Geometry check sheet. Reference: the model listing, model coordinates, mm. Face numbers are marked on the shaded views. Coordinates: 2 decimals unless noted, no trailing zeros. Write item = value, one per line. Start each with the question number.
from build123d import *
from OCP.BRepFilletAPI import BRepFilletAPI_MakeChamfer

# Parameters (mm, degrees)
SKETCH1_R           = 5.25
BOSS_EXTRUDE1_DEPTH = 20
SKETCH1_3_R         = 1.5
BOSS_EXTRUDE2_DEPTH = 17
FILLET1_R           = 15
CHAMFER1_SIZE       = 8.660254038
CHAMFER1_SIZE_2     = 5


with BuildPart() as part:
    # Sketch1 → Boss-Extrude1 (new body)
    # profile 1 of 7: a face of its own
    with BuildSketch(Plane(origin=(0, 0, 0), x_dir=(1, 0, 0), z_dir=(0, 1, 0))):
        with BuildLine():
            Line((-17.320508076, 0), (-12.990381057, 7.5))
            ThreePointArc((-12.990381057, 7.5), (-25.980762114, 0), (-12.990381057, -7.5))
            Line((-12.990381057, -7.5), (-17.320508076, 0))
        make_face()
    # profile 2 of 7: a face of its own
    with BuildSketch(Plane(origin=(0, 0, 0), x_dir=(1, 0, 0), z_dir=(0, 1, 0))):
        Polygon((17.320508076, 0), (8.660254038, 15), (-8.660254038, 15), (-17.320508076, 0), (-8.660254038, -15), (8.660254038, -15), align=None)
        with Locations(Location((0, 0, 0), (0, 0, 270))):
            Circle(SKETCH1_R, mode=Mode.SUBTRACT)
        Polygon((1.443375673, -5.5), (-1.443375673, -5.5), (-2.886751346, -8), (-1.443375673, -10.5), (1.443375673, -10.5), (2.886751346, -8), align=None, mode=Mode.SUBTRACT)
        Polygon((8, 2.886751346), (5.5, 1.443375673), (5.5, -1.443375673), (8, -2.886751346), (10.5, -1.443375673), (10.5, 1.443375673), align=None, mode=Mode.SUBTRACT)
        Polygon((2.886751346, 8), (1.443375673, 10.5), (-1.443375673, 10.5), (-2.886751346, 8), (-1.443375673, 5.5), (1.443375673, 5.5), align=None, mode=Mode.SUBTRACT)
        Polygon((-8, 2.886751346), (-10.5, 1.443375673), (-10.5, -1.443375673), (-8, -2.886751346), (-5.5, -1.443375673), (-5.5, 1.443375673), align=None, mode=Mode.SUBTRACT)
    # profile 3 of 7: a face of its own
    with BuildSketch(Plane(origin=(0, 0, 0), x_dir=(1, 0, 0), z_dir=(0, 1, 0))):
        with BuildLine():
            Line((-12.990381057, 7.5), (-8.660254038, 15))
            Line((-8.660254038, 15), (0, 15))
            ThreePointArc((0, 15), (-12.990381057, 22.5), (-12.990381057, 7.5))
        make_face()
    # profile 4 of 7: a face of its own
    with BuildSketch(Plane(origin=(0, 0, 0), x_dir=(1, 0, 0), z_dir=(0, 1, 0))):
        with BuildLine():
            ThreePointArc((12.990381057, 7.5), (12.990381057, 22.5), (0, 15))
            Line((0, 15), (8.660254038, 15))
            Line((8.660254038, 15), (12.990381057, 7.5))
        make_face()
    # profile 5 of 7: a face of its own
    with BuildSketch(Plane(origin=(0, 0, 0), x_dir=(1, 0, 0), z_dir=(0, 1, 0))):
        with BuildLine():
            ThreePointArc((12.990381057, -7.5), (25.980762114, 0), (12.990381057, 7.5))
            Line((12.990381057, 7.5), (17.320508076, 0))
            Line((17.320508076, 0), (12.990381057, -7.5))
        make_face()
    # profile 6 of 7: a face of its own
    with BuildSketch(Plane(origin=(0, 0, 0), x_dir=(1, 0, 0), z_dir=(0, 1, 0))):
        with BuildLine():
            Line((8.660254038, -15), (0, -15))
            ThreePointArc((0, -15), (12.990381057, -22.5), (12.990381057, -7.5))
            Line((12.990381057, -7.5), (8.660254038, -15))
        make_face()
    # profile 7 of 7: a face of its own
    with BuildSketch(Plane(origin=(0, 0, 0), x_dir=(1, 0, 0), z_dir=(0, 1, 0))):
        with BuildLine():
            Line((-8.660254038, -15), (-12.990381057, -7.5))
            ThreePointArc((-12.990381057, -7.5), (-12.990381057, -22.5), (0, -15))
            Line((0, -15), (-8.660254038, -15))
        make_face()
    extrude(amount=BOSS_EXTRUDE1_DEPTH)

    # Sketch1<3> → Boss-Extrude2 (add)
    # profile 1 of 4: a face of its own
    with BuildSketch(Plane(origin=(0, 0, 0), x_dir=(1, 0, 0), z_dir=(0, 1, 0))):
        Polygon((-8.977463126, 2.322412747), (-10.5, 1.443375673), (-10.5, -1.443375673), (-8.977463126, -2.322412747), (-8, -2.886751346), (-5.5, -1.443375673), (-5.5, 1.443375673), (-8, 2.886751346), align=None)
        with Locations(Location((-8, 0, 0), (0, 0, 90))):
            Circle(SKETCH1_3_R, mode=Mode.SUBTRACT)
    # profile 2 of 4: a face of its own
    with BuildSketch(Plane(origin=(0, 0, 0), x_dir=(1, 0, 0), z_dir=(0, 1, 0))):
        Polygon((2.128194303, 9.313859338), (1.443375673, 10.5), (-1.443375673, 10.5), (-2.128194303, 9.313859338), (-2.886751346, 8), (-1.443375673, 5.5), (1.443375673, 5.5), (2.886751346, 8), align=None)
        with Locations(Location((0, 8, 0), (0, 0, 90))):
            Circle(SKETCH1_3_R, mode=Mode.SUBTRACT)
    # profile 3 of 4: a face of its own
    with BuildSketch(Plane(origin=(0, 0, 0), x_dir=(1, 0, 0), z_dir=(0, 1, 0))):
        Polygon((8, 2.886751346), (5.5, 1.443375673), (5.5, -1.443375673), (8, -2.886751346), (8.977463126, -2.322412747), (10.5, -1.443375673), (10.5, 1.443375673), (8.977463126, 2.322412747), align=None)
        with Locations(Location((8, 0, 0), (0, 0, 90))):
            Circle(SKETCH1_3_R, mode=Mode.SUBTRACT)
    # profile 4 of 4: a face of its own
    with BuildSketch(Plane(origin=(0, 0, 0), x_dir=(1, 0, 0), z_dir=(0, 1, 0))):
        Polygon((1.443375673, -5.5), (-1.443375673, -5.5), (-2.886751346, -8), (-2.128194303, -9.313859338), (-1.443375673, -10.5), (1.443375673, -10.5), (2.128194303, -9.313859338), (2.886751346, -8), align=None)
        with Locations(Location((0, -8, 0), (0, 0, 90))):
            Circle(SKETCH1_3_R, mode=Mode.SUBTRACT)
    extrude(amount=BOSS_EXTRUDE2_DEPTH)

    # Fillet1
    fillet1_edges = [part.edges().sort_by_distance(p)[0] for p in [
        (12.990381057, 10, 7.5),
        (0, 10, 15),
        (-12.990381057, 10, 7.5),
        (-12.990381057, 10, -7.5),
        (0, 10, -15),
        (12.990381057, 10, -7.5),
    ]]
    fillet(fillet1_edges, radius=FILLET1_R)

    # Chamfer1
    chamfer1_edges_1 = [part.edges().sort_by_distance(p)[0] for p in [
        (12.990381057, 20, 22.5),
    ]]
    chamfer1_side_1 = [part.faces().sort_by_distance(p)[0] for p in [
        (12.940381057, 20, 22.41339746),
    ]]
    chamfer1_edges_2 = [part.edges().sort_by_distance(p)[0] for p in [
        (-12.990381057, 20, 22.5),
    ]]
    chamfer1_side_2 = [part.faces().sort_by_distance(p)[0] for p in [
        (-12.940381057, 20, 22.41339746),
    ]]
    chamfer1_edges_3 = [part.edges().sort_by_distance(p)[0] for p in [
        (25.980762114, 20, 0),
    ]]
    chamfer1_side_3 = [part.faces().sort_by_distance(p)[0] for p in [
        (25.880762114, 20, 0),
    ]]
    chamfer1_edges_4 = [part.edges().sort_by_distance(p)[0] for p in [
        (12.990381057, 20, -22.5),
    ]]
    chamfer1_side_4 = [part.faces().sort_by_distance(p)[0] for p in [
        (12.940381057, 20, -22.41339746),
    ]]
    chamfer1_edges_5 = [part.edges().sort_by_distance(p)[0] for p in [
        (-12.990381057, 20, -22.5),
    ]]
    chamfer1_side_5 = [part.faces().sort_by_distance(p)[0] for p in [
        (-12.940381057, 20, -22.41339746),
    ]]
    chamfer1_edges_6 = [part.edges().sort_by_distance(p)[0] for p in [
        (-25.980762114, 20, 0),
    ]]
    chamfer1_side_6 = [part.faces().sort_by_distance(p)[0] for p in [
        (-25.980762114, 19.9, 0),
    ]]
    chamfer1_edges_7 = [part.edges().sort_by_distance(p)[0] for p in [
        (0, 20, 22.018347375),
    ]]
    chamfer1_side_7 = [part.faces().sort_by_distance(p)[0] for p in [
        (0, 20, 21.918347375),
    ]]
    chamfer1_edges_8 = [part.edges().sort_by_distance(p)[0] for p in [
        (19.068448176, 20, 11.009173688),
    ]]
    chamfer1_side_8 = [part.faces().sort_by_distance(p)[0] for p in [
        (18.981845636, 20, 10.959173688),
    ]]
    chamfer1_edges_9 = [part.edges().sort_by_distance(p)[0] for p in [
        (19.068448176, 20, -11.009173688),
    ]]
    chamfer1_side_9 = [part.faces().sort_by_distance(p)[0] for p in [
        (18.981845636, 20, -10.959173688),
    ]]
    chamfer1_edges_10 = [part.edges().sort_by_distance(p)[0] for p in [
        (0, 20, -22.018347375),
    ]]
    chamfer1_side_10 = [part.faces().sort_by_distance(p)[0] for p in [
        (0, 20, -21.918347375),
    ]]
    chamfer1_edges_11 = [part.edges().sort_by_distance(p)[0] for p in [
        (-19.068448176, 20, -11.009173688),
    ]]
    chamfer1_side_11 = [part.faces().sort_by_distance(p)[0] for p in [
        (-19.068448176, 19.9, -11.009173688),
    ]]
    chamfer1_edges_12 = [part.edges().sort_by_distance(p)[0] for p in [
        (-19.068448176, 20, 11.009173688),
    ]]
    chamfer1_side_12 = [part.faces().sort_by_distance(p)[0] for p in [
        (-19.068448176, 19.9, 11.009173688),
    ]]
    chamfer1 = BRepFilletAPI_MakeChamfer(part.part.solid().wrapped)
    for e in chamfer1_edges_1:
        chamfer1.Add(CHAMFER1_SIZE - 0.0001, CHAMFER1_SIZE_2 - 0.0001, e.wrapped, chamfer1_side_1[0].wrapped)
    for e in chamfer1_edges_2:
        chamfer1.Add(CHAMFER1_SIZE - 0.0001, CHAMFER1_SIZE_2 - 0.0001, e.wrapped, chamfer1_side_2[0].wrapped)
    for e in chamfer1_edges_3:
        chamfer1.Add(CHAMFER1_SIZE - 0.0001, CHAMFER1_SIZE_2 - 0.0001, e.wrapped, chamfer1_side_3[0].wrapped)
    for e in chamfer1_edges_4:
        chamfer1.Add(CHAMFER1_SIZE - 0.0001, CHAMFER1_SIZE_2 - 0.0001, e.wrapped, chamfer1_side_4[0].wrapped)
    for e in chamfer1_edges_5:
        chamfer1.Add(CHAMFER1_SIZE - 0.0001, CHAMFER1_SIZE_2 - 0.0001, e.wrapped, chamfer1_side_5[0].wrapped)
    for e in chamfer1_edges_6:
        chamfer1.Add(CHAMFER1_SIZE_2 - 0.0001, CHAMFER1_SIZE - 0.0001, e.wrapped, chamfer1_side_6[0].wrapped)
    for e in chamfer1_edges_7:
        chamfer1.Add(CHAMFER1_SIZE - 0.0001, CHAMFER1_SIZE_2 - 0.0001, e.wrapped, chamfer1_side_7[0].wrapped)
    for e in chamfer1_edges_8:
        chamfer1.Add(CHAMFER1_SIZE - 0.0001, CHAMFER1_SIZE_2 - 0.0001, e.wrapped, chamfer1_side_8[0].wrapped)
    for e in chamfer1_edges_9:
        chamfer1.Add(CHAMFER1_SIZE - 0.0001, CHAMFER1_SIZE_2 - 0.0001, e.wrapped, chamfer1_side_9[0].wrapped)
    for e in chamfer1_edges_10:
        chamfer1.Add(CHAMFER1_SIZE - 0.0001, CHAMFER1_SIZE_2 - 0.0001, e.wrapped, chamfer1_side_10[0].wrapped)
    for e in chamfer1_edges_11:
        chamfer1.Add(CHAMFER1_SIZE_2 - 0.0001, CHAMFER1_SIZE - 0.0001, e.wrapped, chamfer1_side_11[0].wrapped)
    for e in chamfer1_edges_12:
        chamfer1.Add(CHAMFER1_SIZE_2 - 0.0001, CHAMFER1_SIZE - 0.0001, e.wrapped, chamfer1_side_12[0].wrapped)
    add(Compound.cast(chamfer1.Shape()), mode=Mode.REPLACE)  # a hair under: the kernel refuses the full size


solid = part.part
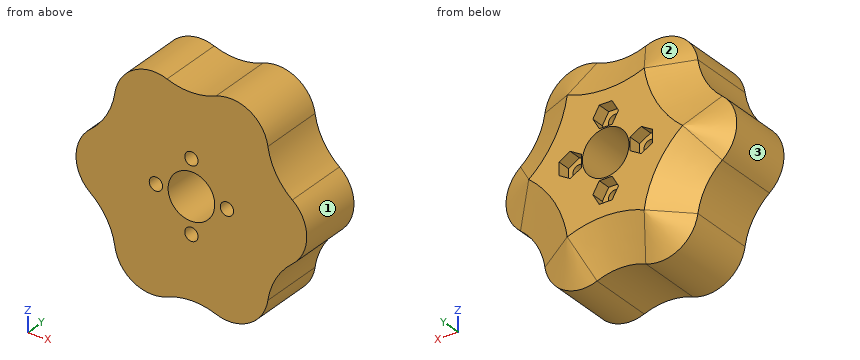
(1) Sectioned sample at A-A on x = 0. Count the separate pieces of the cut face and the enclosed holes in it, plus the area to 3 significant figures.
(2) Draft check along X on the marked faces 1, 2 and 3. Enter one of: pulls with the +X half, pulls with the -X half, needs draft (parallel to the pull), parting line crosses it, or undercut.
(3) Scan lines: line 1 (X direction, y = 5.5, z = 0); line 2 (X direction, y = 9.5, z = 3); line 3 (Z direction, x = -8, y = 12). Record each from-to range of solid material in increasing order.
(4) Depth check by flat-ended pin: pin 1 (4 mm diameter, centred on x = 0, z = -8, fed in from -Y); pin 2 (0.9 mm diameter, centred on y = 18.5, z = -0.5, fed in from -X); pin 3 (1.4 mm diameter, centred on y = 18, z = 0, fed in from -X); pin 4 (6 mm diameter, centred on y = 4.5, z = -6.5, fed in from +X). Enter the tip coordinate at first touch or a pass-through.
Working result:
q1.separate_pieces = 4
q1.enclosed_holes = 0
q1.area = 495 mm2
q2.face_1 = pulls with the +X half
q2.face_2 = undercut
q2.face_3 = pulls with the -X half
q3.line_1 = -25.98 to -9.5, -6.5 to -5.25, 5.25 to 6.5, 9.5 to 25.98
q3.line_2 = -25.44 to -4.31, 4.31 to 25.44
q3.line_3 = -23.64 to -1.5, 1.5 to 23.64
q4.pin_1 = 0
q4.pin_2 = -20.66
q4.pin_3 = -22
q4.pin_4 = 25.24
